Here's how the part is built. I have some questions about the finished solid (model axes, mm). Face numbers are marked on the shaded views. A direction names the side the tool comes from. Give positions to 0.01 mm unless a question says otherwise; leave off trailing zeros. Order: outer loops, then holes, each group sorted by start corner. A loop starts at its lowest first (then second) coordinate and runs counter-clockwise, first axis right, second up.
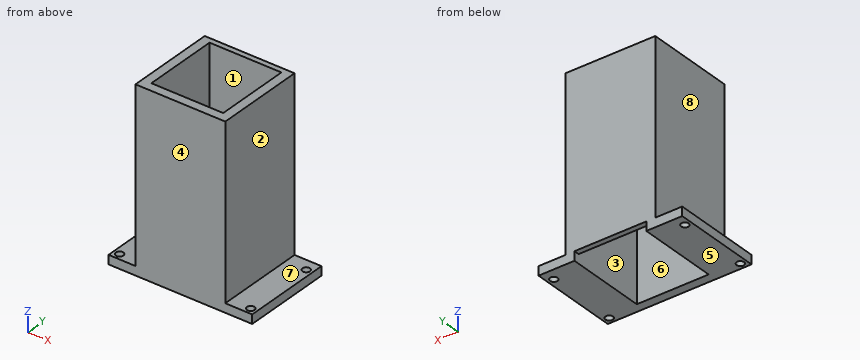
from build123d import *

# Parameters (mm, degrees)
SKETCH_1_W          = 80
SKETCH_1_H          = 50
EXTRUDE_1_DEPTH     = 5
SKETCH_2_W          = 50
SKETCH_2_H          = 50
EXTRUDE_2_DEPTH     = 100
SKETCH_4_W          = 40
SKETCH_4_H          = 42
CUT_EXTRUDE_1_DEPTH = 138.477270849
SKETCH_5_R          = 2.1
CUT_EXTRUDE_2_DEPTH = 10
CUT_EXTRUDE_START   = 40
SKETCH_7_W          = 40
SKETCH_7_H          = 5
CUT_EXTRUDE_4_DEPTH = 98.477270849


with BuildPart() as part:
    # 草圖1 → 填料-伸長1 (new body)
    with BuildSketch(Plane.XY):
        with Locations((40, 25)):
            Rectangle(SKETCH_1_W, SKETCH_1_H)
    extrude(amount=EXTRUDE_1_DEPTH)

    # 草圖2 → 填料-伸長2 (add)
    with BuildSketch(Plane.XY):
        with Locations((40, 25)):
            Rectangle(SKETCH_2_W, SKETCH_2_H)
    extrude(amount=EXTRUDE_2_DEPTH)

    # 草圖4 → 除料-伸長1 (cut, through all)
    with BuildSketch(Plane.XY):
        with Locations((40, 26)):
            Rectangle(SKETCH_4_W, SKETCH_4_H)
    extrude(amount=CUT_EXTRUDE_1_DEPTH, mode=Mode.SUBTRACT)

    # 草圖5 → 除料-伸長2 (cut)
    with BuildSketch(Plane.XY):
        with Locations(Location((76.5, 3.5, 0), (0, 0, 180))):
            Circle(SKETCH_5_R)
        with Locations(Location((76.5, 43.5, 0), (0, 0, 180))):
            Circle(SKETCH_5_R)
        with Locations(Location((3.5, 3.5, 0), (0, 0, 180))):
            Circle(SKETCH_5_R)
        with Locations(Location((3.5, 43.5, 0), (0, 0, 180))):
            Circle(SKETCH_5_R)
    extrude(amount=CUT_EXTRUDE_2_DEPTH, mode=Mode.SUBTRACT)

    # 草圖7 → 除料-伸長4 (cut, through all)
    with BuildSketch(Plane(origin=(0, 0, 0), x_dir=(1, 0, 0), z_dir=(0, 1, 0)).offset(CUT_EXTRUDE_START)):
        with Locations((40, -2.5)):
            Rectangle(SKETCH_7_W, SKETCH_7_H)
    extrude(amount=CUT_EXTRUDE_4_DEPTH, mode=Mode.SUBTRACT)


solid = part.part
Q1. If we section it at A-A on y = 3.5: List the corners of the cut face in (x, z) for me, plus the area to 3 significant figures.
Filled sheet:
outline: (0, 0) - (1.4, 0) - (1.4, 5) - (0, 5) - close; (5.6, 0) - (74.4, 0) - (74.4, 5) - (65, 5) - (65, 100) - (15, 100) - (15, 5) - (5.6, 5) - close; (78.6, 0) - (80, 0) - (80, 5) - (78.6, 5) - close
area: 5,110 mm2
Q2. If we section it at C-C on y = 43.5: List the corners of the cut face in (x, z) for me.
Filled sheet:
outline: (0, 0) - (1.4, 0) - (1.4, 5) - (0, 5) - close; (5.6, 0) - (20, 0) - (20, 100) - (15, 100) - (15, 5) - (5.6, 5) - close; (60, 0) - (74.4, 0) - (74.4, 5) - (65, 5) - (65, 100) - (60, 100) - close; (78.6, 0) - (80, 0) - (80, 5) - (78.6, 5) - close
Q3. I need wall thicknesses on L1, parallel to Y at x = 3.5, z = 3.55; L2, parallel to X at y = 43.5, z = 3.05; L3, parallel to X at y = 46, z = 49.5. Which ranges of each line are inside material? Lowest first, please.
Filled sheet:
L1: y = 0 to 1.4, 5.6 to 41.4, 45.6 to 50
L2: x = 0 to 1.4, 5.6 to 20, 60 to 74.4, 78.6 to 80
L3: x = 15 to 20, 60 to 65
Q4. I'm going to push flat-ended pins straight in: P1, Ø7.5, axis at x = 69.5, y = 33.5, coming from the +Z side; P2, Ø25, axis at y = 16, z = 63.5, coming from the +X side; P3, Ø2.5, axis at x = 33, y = 48, coming from the -Z side; P4, Ø12, axis at x = 42, z = 60.5, coming from the -Y side. Where does each tip first touch, or does it pass through?
Filled sheet:
P1: stops at z = 5
P2: stops at x = 65
P3: stops at z = 5
P4: stops at y = 0
Q5. Thinking about a two-plate mould opening in X: for the marked faces 1, 2, 3 and 4, which applies, released by +X, released by -X, zero draft, split by the parting line, or undercut?
Filled sheet:
face 1: undercut
face 2: released by +X
face 3: undercut
face 4: zero draft
Q6. For the marked faces 5, 6, 7 and 8, which set-ups out of +Z, -Z, +X, -X, +Y, -Y let a thin tool reach every point of the face, with its end or its side?
Filled sheet:
face 5: -Z, +X, -X, +Y, -Y
face 6: +Z, -Z
face 7: +Z, +X, +Y, -Y
face 8: +Z, -X, +Y, -Y
Q7. If we section it at B-B on x = 32: List the corners of the cut face in (y, z) for me, plus the area to 3 significant figures.
Filled sheet:
outline: (0, 0) - (5, 0) - (5, 100) - (0, 100) - close; (47, 5) - (50, 5) - (50, 100) - (47, 100) - close
area: 785 mm2
Q8. If we section it at D-D on z = 83: List the corners of the cut face in (x, y) for me.
Filled sheet:
outline: (15, 0) - (65, 0) - (65, 50) - (15, 50) - close; hole (20, 5) - (60, 5) - (60, 47) - (20, 47) - close
